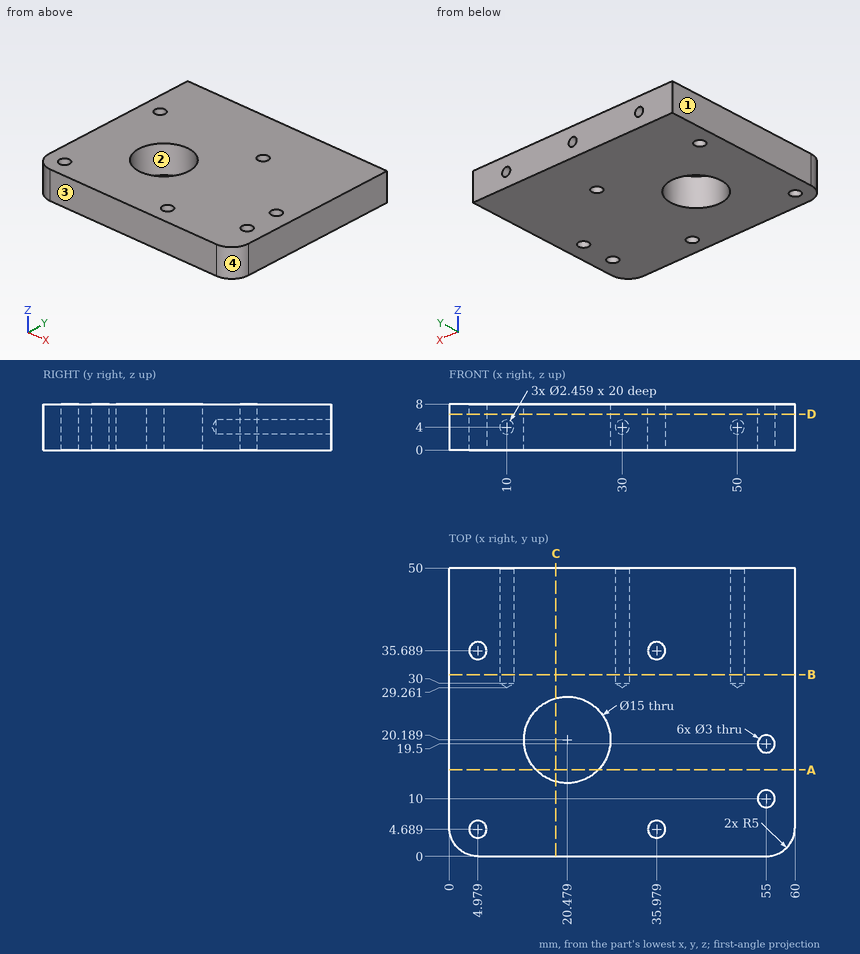
Can you work these out from the drawing? Everything is in mm from the part's minimum corner. Coordinates: 2 decimals unless noted, no trailing zeros. Loops run counter-clockwise (first coordinate to the right, second up) from the corner with the lowest first, then second, coordinate; pieces in that order, holes last.
1) Imagine slicing it at D-D on z = 6.25. List the corners of the cut face in (x, y) for me, plus the area to 3 significant figures.
2) I need wall thicknesses on probe 1 along X at (y, z) = (41, 4); probe 2 along X at (y, z) = (3.5, 4) (1 decimal); probe 3 along Y at (x, z) = (55, 6). Which ranges of each line are inside material? Lowest first, please.
3) For pin 1 (1.8 mm diameter, centred on x = 35.98, y = 4.69, fed in from +Z); pin 2 (4 mm diameter, centred on x = 55, y = 19.5, fed in from +Z); pin 3 (2 mm diameter, centred on x = 10, z = 4, fed in from +Y), each with a flat end and sliding along its axis, tell me the tip position at first contact or that it passes through.
4) Imagine slicing it at B-B on y = 31.5. List the corners of the cut face in (x, z) for me, plus the area to 3 significant figures.
5) Thinking about a two-plate mould opening in X: for the marked faces 1, 2, 3 and 4, which applies, pulls with the +X half, pulls with the -X half, needs draft (parallel to the pull), parting line crosses it, or undercut?
6) Imagine slicing it at A-A on y = 15. List the corners of the cut face in (x, z) for me.
7) Imagine slicing it at C-C on x = 18.5. List the corners of the cut face in (y, z) for me (1 decimal), plus the area to 3 significant figures.
Completed:
1. outline: (0, 5) arc R5 ccw to (5, 0) - (55, 0) arc R5 ccw to (60, 5) - (60, 50) - (0, 50) - close; hole circle Ø3 at (4.98, 4.69); hole circle Ø3 at (4.98, 35.69); hole circle Ø15 at (20.48, 20.19); hole circle Ø3 at (35.98, 4.69); hole circle Ø3 at (35.98, 35.69); hole circle Ø3 at (55, 10); hole circle Ø3 at (55, 19.5)
1. area: 2,770 mm2
2. probe 1: x = 0 to 8.77, 11.23 to 28.77, 31.23 to 48.77, 51.23 to 60
2. probe 2: x = 0.2 to 4.1, 5.9 to 35.1, 36.9 to 59.8
2. probe 3: y = 0 to 8.5, 11.5 to 18, 21 to 50
3. pin 1: passes through
3. pin 2: stops at z = 8
3. pin 3: stops at y = 29.86
4. outline: (0, 0) - (60, 0) - (60, 8) - (0, 8) - close; hole circle Ø2.46 at (10, 4); hole circle Ø2.46 at (30, 4); hole circle Ø2.46 at (50, 4)
4. area: 466 mm2
5. face 1: pulls with the -X half
5. face 2: undercut
5. face 3: needs draft
5. face 4: pulls with the +X half
6. outline: (0, 0) - (15.06, 0) - (15.06, 8) - (0, 8) - close; (25.89, 0) - (60, 0) - (60, 8) - (25.89, 8) - close
7. outline: (0, 0) - (13, 0) - (13, 8) - (0, 8) - close; (27.4, 0) - (50, 0) - (50, 8) - (27.4, 8) - close
7. area: 284 mm2
